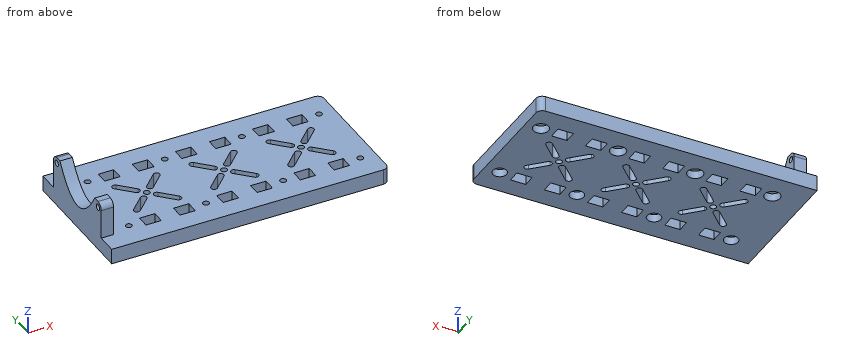
from build123d import *

# Parameters (mm, degrees)
IZIM1_W                     = 180
IZIM1_H                     = 85
Y_KSEKLIK_EKSTR_ZYON1_DEPTH = 10
IZIM2_R                     = 2
IZIM2_W                     = 10
IZIM2_H                     = 8
KES_EKSTR_ZYON1_DEPTH       = 10
IZIM3_R                     = 5
IZIM3_R_2                   = 4.5
KES_EKSTR_ZYON2_DEPTH       = 5
SKETCH1_R                   = 2
BOSS_EXTRUDE1_DEPTH         = 8
FILLET1_R                   = 4


with BuildPart() as part:
    # Çizim1 → Yükseklik-Ekstrüzyon1 (new body)
    with BuildSketch(Plane.XY):
        Rectangle(IZIM1_W, IZIM1_H)
    extrude(amount=Y_KSEKLIK_EKSTR_ZYON1_DEPTH)

    # Çizim2 → Kes-Ekstrüzyon1 (cut)
    with BuildSketch(Plane.XY.offset(10)):
        with Locations((-70, -25.5)):
            Circle(IZIM2_R)
        with Locations((-45, 0)):
            Circle(IZIM2_R)
        with Locations((-70, 25.5)):
            Circle(IZIM2_R)
        with Locations((80, 25.5)):
            Circle(IZIM2_R)
        with Locations((80, -25.5)):
            Circle(IZIM2_R)
        with Locations((-20, 25.5)):
            Circle(IZIM2_R)
        with Locations((5, 0)):
            Circle(IZIM2_R)
        with Locations((-20, -25.5)):
            Circle(IZIM2_R)
        with Locations((30, 25.5)):
            Circle(IZIM2_R)
        with Locations((55, 0)):
            Circle(IZIM2_R)
        with Locations((30, -25.5)):
            Circle(IZIM2_R)
        with Locations((-56, -25.5)):
            Rectangle(IZIM2_W, IZIM2_H)
        with BuildLine():
            Line((-59.849242405, -12.02081528), (-50.656854249, -2.828427125))
            ThreePointArc((-50.656854249, -2.828427125), (-47.828427125, -2.828427125), (-47.828427125, -5.656854249))
            Line((-47.828427125, -5.656854249), (-57.02081528, -14.849242405))
            ThreePointArc((-57.02081528, -14.849242405), (-59.849242405, -14.849242405), (-59.849242405, -12.02081528))
        make_face()
        with Locations((-34, -25.5)):
            Rectangle(IZIM2_W, IZIM2_H)
        with BuildLine():
            Line((-30.150757595, -12.02081528), (-39.343145751, -2.828427125))
            ThreePointArc((-39.343145751, -2.828427125), (-42.171572875, -2.828427125), (-42.171572875, -5.656854249))
            Line((-42.171572875, -5.656854249), (-32.97918472, -14.849242405))
            ThreePointArc((-32.97918472, -14.849242405), (-30.150757595, -14.849242405), (-30.150757595, -12.02081528))
        make_face()
        with BuildLine():
            Line((-59.849242405, 12.02081528), (-50.656854249, 2.828427125))
            ThreePointArc((-50.656854249, 2.828427125), (-47.828427125, 2.828427125), (-47.828427125, 5.656854249))
            Line((-47.828427125, 5.656854249), (-57.02081528, 14.849242405))
            ThreePointArc((-57.02081528, 14.849242405), (-59.849242405, 14.849242405), (-59.849242405, 12.02081528))
        make_face()
        with BuildLine():
            Line((-30.150757595, 12.02081528), (-39.343145751, 2.828427125))
            ThreePointArc((-39.343145751, 2.828427125), (-42.171572875, 2.828427125), (-42.171572875, 5.656854249))
            Line((-42.171572875, 5.656854249), (-32.97918472, 14.849242405))
            ThreePointArc((-32.97918472, 14.849242405), (-30.150757595, 14.849242405), (-30.150757595, 12.02081528))
        make_face()
        with Locations((-34, 25.5)):
            Rectangle(IZIM2_W, IZIM2_H)
        with Locations((-56, 25.5)):
            Rectangle(IZIM2_W, IZIM2_H)
        with Locations((-6, 25.5)):
            Rectangle(IZIM2_W, IZIM2_H)
        with Locations((16, 25.5)):
            Rectangle(IZIM2_W, IZIM2_H)
        with BuildLine():
            Line((-9.849242405, 12.02081528), (-0.656854249, 2.828427125))
            ThreePointArc((-0.656854249, 2.828427125), (2.171572875, 2.828427125), (2.171572875, 5.656854249))
            Line((2.171572875, 5.656854249), (-7.02081528, 14.849242405))
            ThreePointArc((-7.02081528, 14.849242405), (-9.849242405, 14.849242405), (-9.849242405, 12.02081528))
        make_face()
        with BuildLine():
            Line((19.849242405, 12.02081528), (10.656854249, 2.828427125))
            ThreePointArc((10.656854249, 2.828427125), (7.828427125, 2.828427125), (7.828427125, 5.656854249))
            Line((7.828427125, 5.656854249), (17.02081528, 14.849242405))
            ThreePointArc((17.02081528, 14.849242405), (19.849242405, 14.849242405), (19.849242405, 12.02081528))
        make_face()
        with BuildLine():
            Line((17.02081528, -14.849242405), (7.828427125, -5.656854249))
            ThreePointArc((7.828427125, -5.656854249), (7.828427125, -2.828427125), (10.656854249, -2.828427125))
            Line((10.656854249, -2.828427125), (19.849242405, -12.02081528))
            ThreePointArc((19.849242405, -12.02081528), (19.849242405, -14.849242405), (17.02081528, -14.849242405))
        make_face()
        with BuildLine():
            Line((-9.849242405, -12.02081528), (-0.656854249, -2.828427125))
            ThreePointArc((-0.656854249, -2.828427125), (2.171572875, -2.828427125), (2.171572875, -5.656854249))
            Line((2.171572875, -5.656854249), (-7.02081528, -14.849242405))
            ThreePointArc((-7.02081528, -14.849242405), (-9.849242405, -14.849242405), (-9.849242405, -12.02081528))
        make_face()
        with Locations((-6, -25.5)):
            Rectangle(IZIM2_W, IZIM2_H)
        with Locations((16, -25.5)):
            Rectangle(IZIM2_W, IZIM2_H)
        with Locations((44, 25.5)):
            Rectangle(IZIM2_W, IZIM2_H)
        with Locations((66, 25.5)):
            Rectangle(IZIM2_W, IZIM2_H)
        with BuildLine():
            Line((40.150757595, 12.02081528), (49.343145751, 2.828427125))
            ThreePointArc((49.343145751, 2.828427125), (52.171572875, 2.828427125), (52.171572875, 5.656854249))
            Line((52.171572875, 5.656854249), (42.97918472, 14.849242405))
            ThreePointArc((42.97918472, 14.849242405), (40.150757595, 14.849242405), (40.150757595, 12.02081528))
        make_face()
        with BuildLine():
            Line((69.849242405, 12.02081528), (60.656854249, 2.828427125))
            ThreePointArc((60.656854249, 2.828427125), (57.828427125, 2.828427125), (57.828427125, 5.656854249))
            Line((57.828427125, 5.656854249), (67.02081528, 14.849242405))
            ThreePointArc((67.02081528, 14.849242405), (69.849242405, 14.849242405), (69.849242405, 12.02081528))
        make_face()
        with BuildLine():
            Line((67.02081528, -14.849242405), (57.828427125, -5.656854249))
            ThreePointArc((57.828427125, -5.656854249), (57.828427125, -2.828427125), (60.656854249, -2.828427125))
            Line((60.656854249, -2.828427125), (69.849242405, -12.02081528))
            ThreePointArc((69.849242405, -12.02081528), (69.849242405, -14.849242405), (67.02081528, -14.849242405))
        make_face()
        with BuildLine():
            Line((40.150757595, -12.02081528), (49.343145751, -2.828427125))
            ThreePointArc((49.343145751, -2.828427125), (52.171572875, -2.828427125), (52.171572875, -5.656854249))
            Line((52.171572875, -5.656854249), (42.97918472, -14.849242405))
            ThreePointArc((42.97918472, -14.849242405), (40.150757595, -14.849242405), (40.150757595, -12.02081528))
        make_face()
        with Locations((44, -25.5)):
            Rectangle(IZIM2_W, IZIM2_H)
        with Locations((66, -25.5)):
            Rectangle(IZIM2_W, IZIM2_H)
    extrude(amount=-KES_EKSTR_ZYON1_DEPTH, mode=Mode.SUBTRACT)

    # Çizim3 → Kes-Ekstrüzyon2 (cut)
    with BuildSketch(Plane(origin=(0, 0, 0), x_dir=(-1, 0, 0), z_dir=(0, 0, -1))):
        with Locations((70, 25.5)):
            Circle(IZIM3_R)
        with Locations((70, -25.5)):
            Circle(IZIM3_R_2)
        with Locations((20, 25.5)):
            Circle(IZIM3_R)
        with Locations((20, -25.5)):
            Circle(IZIM3_R_2)
        with Locations((-30, 25.5)):
            Circle(IZIM3_R)
        with Locations((-30, -25.5)):
            Circle(IZIM3_R_2)
        with Locations((-80, 25.5)):
            Circle(IZIM3_R)
        with Locations((-80, -25.5)):
            Circle(IZIM3_R_2)
    extrude(amount=-KES_EKSTR_ZYON2_DEPTH, mode=Mode.SUBTRACT)

    # Sketch1 → Boss-Extrude1 (add)
    with BuildSketch(Plane.ZY.offset(90)):
        with BuildLine():
            Line((10, -29.5), (33, -29.5))
            Line((33, -29.5), (33, -21.5))
            add(Edge.make_bspline(
                [(33, 21.5), (-3, 0), (33, -21.5)],
                knots=[0, 0, 0, 1, 1, 1], degree=2))
            Line((33, 21.5), (33, 29.5))
            Line((33, 29.5), (10, 29.5))
            Line((10, 29.5), (10, -29.5))
        make_face()
        with Locations((29, -25.5)):
            Circle(SKETCH1_R, mode=Mode.SUBTRACT)
        with Locations((29, 25.5)):
            Circle(SKETCH1_R, mode=Mode.SUBTRACT)
    extrude(amount=-BOSS_EXTRUDE1_DEPTH)

    # Fillet1
    fillet1_edges = [part.edges().sort_by_distance(p)[0] for p in [
        (-86, 29.5, 33),
        (-86, -29.5, 33),
        (90, 42.5, 5),
        (90, -42.5, 5),
    ]]
    fillet(fillet1_edges, radius=FILLET1_R)


solid = part.part
Part model, mm, in its own coordinate system. Coordinates: 2 decimals unless noted, no trailing zeros. Loops run counter-clockwise (first coordinate to the right, second up) from the corner with the lowest first, then second, coordinate; pieces in that order, holes last. Notation, with made-up numbers: (-0.75, 75.25) -> (44.25, 75.25) arc R14 cw to (44.25, 87.25) -> close; hole circle Ø5 at (38.5, 34.5). An arc over 180 degrees is marked (long way). Use a Markdown table: item, result. Add a question column.
Item 1: Band-saw the part on B-B on x = -20. Write the cut outline in (y, z).
Item 2: Flat gauge pins, fed straight in: P1, Ø8, axis at x = 80, y = -25.5, coming from the +Z side; P2, Ø3, axis at x = -20.5, y = 24, coming from the -Z side; P3, Ø2.5, axis at x = -88, z = 21, coming from the +Y side. Where does each tip first touch, or does it go through?
Item 3: Band-saw the part on A-A on x = 5. Write the cut outline in (y, z), plus the area to 3 significant figures.
Item 4: Probe probe 1 along Y at (x, z) = (30, 8); probe 2 along Y at (x, z) = (30, 2.5); probe 3 along Y at (x, z) = (-85, 29). List the from-to ranges inside material, lowest first.
Item 5: Band-saw the part on C-C on y = 0. Give the number of separate pieces and of enclosed holes in the cut face, plus the area to 3 significant figures.
Geometry says:
| question | item | result |
|---|---|---|
| 1 | outline | (-42.5, 0) -> (-30, 0) -> (-30, 5) -> (-27.5, 5) -> (-27.5, 10) -> (-42.5, 10) -> close; (-23.5, 5) -> (-21, 5) -> (-21, 0) -> (20.5, 0) -> (20.5, 5) -> (23.5, 5) -> (23.5, 10) -> (-23.5, 10) -> close; (27.5, 5) -> (30.5, 5) -> (30.5, 0) -> (42.5, 0) -> (42.5, 10) -> (27.5, 10) -> close |
| 2 | P1 | z = 10 |
| 2 | P2 | z = 5 |
| 2 | P3 | y = 29.5 |
| 3 | outline | (-42.5, 0) -> (-2, 0) -> (-2, 10) -> (-42.5, 10) -> close; (2, 0) -> (42.5, 0) -> (42.5, 10) -> (2, 10) -> close |
| 3 | area | 810 mm² |
| 4 | probe 1 | -42.5 to -27.5, -23.5 to 23.5, 27.5 to 42.5 |
| 4 | probe 2 | -42.5 to -30, -21 to 20.5, 30.5 to 42.5 |
| 4 | probe 3 | -29.5 to -27.5, -23.5 to -18.96, 18.96 to 23.5, 27.5 to 29.5 |
| 5 | separate pieces | 4 |
| 5 | enclosed holes | 0 |
| 5 | area | 1,720 mm² |
